```python
from build123d import *

# Parameters (mm, degrees)
SKETCH_W        = 50
SKETCH_H        = 6
PAD_DEPTH       = 5
SKETCH001_R     = 1.6
POCKET_DEPTH    = 5
POCKET001_DEPTH = 2


with BuildPart() as part:
    # Sketch → Pad (new body)
    with BuildSketch(Plane.XY):
        with Locations((25, 3)):
            Rectangle(SKETCH_W, SKETCH_H)
    extrude(amount=PAD_DEPTH)

    # Sketch001 (on Face6 of Pad) → Pocket (cut)
    with BuildSketch(Plane.XY.offset(5)):
        with Locations((12.5, 3)):
            Circle(SKETCH001_R)
        with Locations((37.5, 3)):
            Circle(SKETCH001_R)
    extrude(amount=-POCKET_DEPTH, mode=Mode.SUBTRACT)

    # Sketch002 (on Face5 of Pocket) → Pocket001 (cut)
    with BuildSketch(Plane.XY.offset(5)):
        Polygon((15.25, 4.587713), (12.5, 6.175426), (9.75, 4.587713), (9.75, 1.412287), (12.5, -0.175426), (15.25, 1.412287), align=None)
        Polygon((40.25, 1.412287), (40.25, 4.587713), (37.5, 6.175426), (34.75, 4.587713), (34.75, 1.412287), (37.5, -0.175426), align=None)
    extrude(amount=-POCKET001_DEPTH, mode=Mode.SUBTRACT)


solid = part.part
```
Build history of the part. All positions in model axes, mm. A direction names the side the tool comes from. Round coordinates to 2 decimals unless told otherwise and drop trailing zeros. Write each loop counter-clockwise with the first axis right and the second up, starting at its lowest first coordinate (ties: lowest second). Pieces come first, ordered by that corner, then holes. Notation, with made-up numbers: (72, 12) - (120, 12) arc R9 cw to (120, 19) - close; hole circle Ø10 at (-2.75, 56). An arc over 180 degrees is marked (long way). Write each question's results on one line, items separated by ' | '. Start each with the question number.
Item 1: Wall check: L1, parallel to X at y = 2.25, z = 3.05; L2, parallel to Y at x = 12.5, z = 1; L3, parallel to X at y = 2.75, z = 1.2. Give the ranges that are in metal, low to high. Write a range as [from, to].
Item 2: Saw through at A-A (z = 1.5). Write the cut outline in (x, y), and give its area (3 significant figures).
Item 3: Drop flat-ended pins along their axis: P1, Ø3.5, axis at x = 37.5, y = 3, coming from the +Z side; P2, Ø3, axis at x = 12.5, y = 3, coming from the +Z side. Give the stop position or say it passes through.
Item 4: Saw through at B-B (z = 3.7). Write the cut outline in (x, y).
Item 5: Mould opens along X. For faces 3 (the face through (50, 3, 2)), 4 (the face through (38.24, 1.58, 1.52)), 5 (the face through (25, 3, 0)) say: pulls with the +X half, pulls with the -X half, needs draft (parallel to the pull), parting line crosses it, or undercut.
Item 6: Which spindle directions (+Z, -Z, +X, -X, +Y, -Y) get a long thin tool onto all of the face, cutting with end or side? Do faces 1 (the face through (5, 3, 5)), 2 (the face through (9.75, 3, 4)). Say none if no direction does.
Results are:
1) L1: x = [0, 9.75], [15.25, 34.75], [40.25, 50] | L2: y = [0, 1.4], [4.6, 6] | L3: x = [0, 10.92], [14.08, 35.92], [39.08, 50]
2) outline: (0, 0) - (50, 0) - (50, 6) - (0, 6) - close; hole circle Ø3.2 at (12.5, 3); hole circle Ø3.2 at (37.5, 3) | area: 284 mm²
3) P1: stops at z = 3 | P2: passes through
4) outline: (0, 0) - (12.2, 0) - (9.75, 1.41) - (9.75, 4.59) - (12.2, 6) - (0, 6) - close; (12.8, 0) - (37.2, 0) - (34.75, 1.41) - (34.75, 4.59) - (37.2, 6) - (12.8, 6) - (15.25, 4.59) - (15.25, 1.41) - close; (37.8, 0) - (50, 0) - (50, 6) - (37.8, 6) - (40.25, 4.59) - (40.25, 1.41) - close
5) face 3: pulls with the +X half | face 4: undercut | face 5: needs draft
6) face 1: +Z, +X, -X, +Y, -Y | face 2: +Z
